Input: part model. Units: mm. Frame: model coordinates. Give positions to 0.01 mm unless a question says otherwise; leave off trailing zeros. Write each loop counter-clockwise with the first axis right and the second up, starting at its lowest first coordinate (ties: lowest second). Pieces come first, ordered by that corner, then holes. Notation, with made-up numbers: (-36, 72) - (-31, 72) arc R24 cw to (-31, 90) - close; hole circle Ø10 at (21.5, 44.5). An arc over 180 degrees is marked (long way). Use a Markdown table: item, result. Add a question column.
1. Section query D-D, the plane x = 90. Return loops of the section in (y, z), plus the area to 4 significant figures.
2. Section query C-C, the plane z = -10. Return loops of the section in (x, y), plus the area to 3 significant figures.
3. Mould query, pull axis Z, two halves, no side actions, for faces 1 (the flat face through (61, 2, -59)), 2 (the flat face through (100, 2, -10)), 3 (the cylindrical face through (92.747, 2.465, -10.121)), 4 (the flat face through (49, 2, 0)). Classes: released by +Z, released by -Z, zero draft, split by the parting line, or undercut.
4. Section query B-B, the plane x = 10. Return loops of the section in (y, z), plus the area to 4 significant figures.
5. Section query A-A, the plane z = -90. Return loops of the section in (x, y).
6. Material intervals for probe 1 along Z at (x, y) = (10, 3.1); probe 2 along Z at (x, y) = (9, 0.5); probe 3 along X at (y, z) = (1.9, -8), sorted ascending.
7. Pin query (flat end, axial travel): pin 1 (3 mm diameter, centred on y = 3.5, z = -81, fed in from +X); pin 2 (2 mm diameter, centred on x = 55.5, y = 1.5, fed in from -Z). Return the tip coordinate at first contact, or that it passes through.
Autodesk Inventor part; units mm, degrees
ref_plane "YZ Plane" through (0, 0, 0) normal (1, 0, 0) x (0, 1, 0)
ref_plane "XZ Plane" through (0, 0, 0) normal (0, 1, 0) x (-1, 0, 0)
ref_plane "XY Plane" through (0, 0, 0) normal (0, 0, 1) x (1, 0, 0)
sketch "Sketch1" plane through (0, 0, 0) normal (0, 1, 0) x (-1, 0, 0)
  line L0 (0, 0) -> (0, -100)
  line L1 (0, -100) -> (-20, -100)
  line L2 (0, 0) -> (-100, 0)
  line L3 (-100, 0) -> (-100, -20)
  line L4 (-100, -20) -> (-20, -100)
  line L5 (26.0864, -10) -> (-132.7995, -10) construction
  line L6 (-10, 33.7229) -> (-10, -136.0235) construction
  circle A0 centre (-10, -10) radius 2.75
  circle A1 centre (-10, -90) radius 2.75
  circle A2 centre (-10, -30) radius 2.75
  circle A3 centre (-90, -10) radius 2.75
  dimension "d0" = 100
  dimension "d1" = 20
  dimension "d2" = 100
  dimension "d3" = 20
  dimension "d4" = 10
  dimension "d5" = 10
  dimension "d6" = 5.5
  dimension "d7" = 5.5
  dimension "d8" = 5.5
  dimension "d9" = 5.5
  dimension "d10" = 10
  dimension "d11" = 30
  dimension "d12" = 10
extrude "Extrusion1" add sketch "Sketch1" along normal blind 5
equation "\"d0\" = dimension"
equation "\"d1\" = perfil_ancho"
equation "\"d2\" = dimension"
equation "\"d3\" = perfil_ancho"
equation "\"d4\" = 0.5 * perfil_ancho"
equation "\"d5\" = 0.5 * perfil_ancho"
equation "\"d6\" = hueco_diametro"
equation "\"d7\" = hueco_diametro"
equation "\"d8\" = hueco_diametro"
equation "\"d9\" = hueco_diametro"
equation "\"d10\" = separación"
equation "\"d11\" = perfil_ancho + separación"
equation "\"d12\" = separación"
equation "\"d13\" = espesor"
equation "\"perfil_ancho\" = 20"
equation "\"dimension\" = 100"
equation "\"separación\" = 10"
equation "\"espesor\" = 5"
equation "\"tol\" = 0.5"
properties part number "soporte tipo triangulo"
Result sheet:
| question | item | result |
|---|---|---|
| 1 | outline | (0, -30) - (5, -30) - (5, -12.75) - (0, -12.75) - close; (0, -7.25) - (5, -7.25) - (5, 0) - (0, 0) - close |
| 1 | area | 122.5 mm² |
| 2 | outline | (0, 0) - (7.25, 0) - (7.25, 5) - (0, 5) - close; (12.75, 0) - (87.25, 0) - (87.25, 5) - (12.75, 5) - close; (92.75, 0) - (100, 0) - (100, 5) - (92.75, 5) - close |
| 2 | area | 445 mm² |
| 3 | face 1 | released by -Z |
| 3 | face 2 | zero draft |
| 3 | face 3 | undercut |
| 3 | face 4 | released by +Z |
| 4 | outline | (0, -100) - (5, -100) - (5, -92.75) - (0, -92.75) - close; (0, -87.25) - (5, -87.25) - (5, -32.75) - (0, -32.75) - close; (0, -27.25) - (5, -27.25) - (5, -12.75) - (0, -12.75) - close; (0, -7.25) - (5, -7.25) - (5, 0) - (0, 0) - close |
| 4 | area | 417.5 mm² |
| 5 | outline | (0, 0) - (7.25, 0) - (7.25, 5) - (0, 5) - close; (12.75, 0) - (30, 0) - (30, 5) - (12.75, 5) - close |
| 6 | probe 1 | z = -100 to -92.75, -87.25 to -32.75, -27.25 to -12.75, -7.25 to 0 |
| 6 | probe 2 | z = -100 to -92.56, -87.44 to -32.56, -27.44 to -12.56, -7.44 to 0 |
| 6 | probe 3 | x = 0 to 8.11, 11.89 to 88.11, 91.89 to 100 |
| 7 | pin 1 | stops at x = 40.5 |
| 7 | pin 2 | stops at z = -65.5 |
